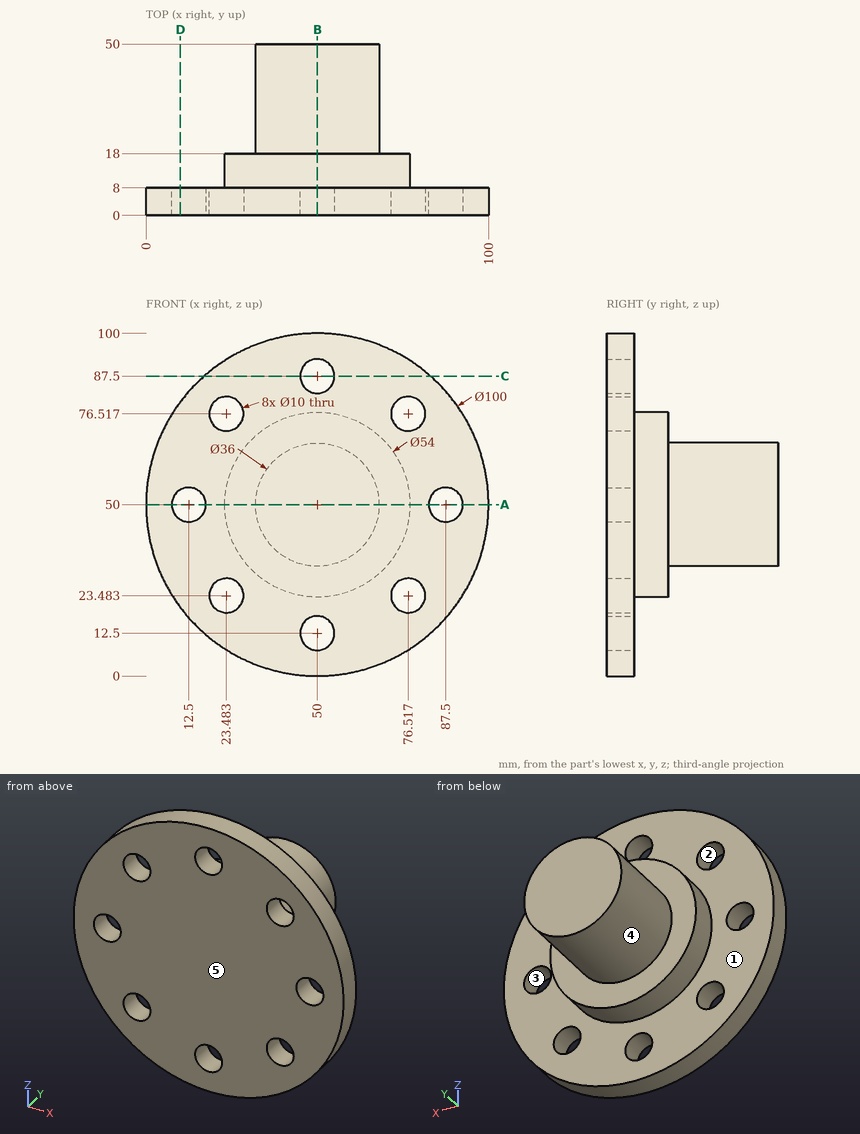
Could you check a few things on this drawing? It's one solid part, dimensions in mm from its lowest x, y, z. A direction names the side the tool comes from. Round coordinates to 2 decimals unless told otherwise and drop trailing zeros. Order: outer loops, then holes, each group sorted by start corner. A loop starts at its lowest first (then second) coordinate and runs counter-clockwise, first axis right, second up. Notation, with made-up numbers: (11.5, 38.5) -> (45.5, 38.5) arc R24 cw to (45.5, 61.5) -> close; hole circle Ø2 at (-24.5, 63.5). An arc over 180 degrees is marked (long way). One line per question, with ' | ' between items.
Q1. We'd pull the mould along X, two halves only. Please class the marked faces 3, 4 and 5: released by +X, released by -X, zero draft, split by the parting line, or undercut.
Computed values:
face 3: undercut | face 4: split by the parting line | face 5: zero draft
Q2. If I drill on line 1 (Y direction, x = 10.5, z = 31); line 2 (Z direction, x = 73, y = 7.5) (1 decimal); line 3 (X direction, y = 5, z = 74.5) (1 decimal), over which ranges is the centre line in solid material (lowest first)? Write a range as from..to.
Computed values:
line 1: 0..8 | line 2: 5.6..19.9, 27..73, 80.1..94.4 | line 3: 6.4..18.9, 28.1..71.9, 81.1..93.6
Q3. Which directions (+Z, -Z, +X, -X, +Y, -Y) give clear straight access to the entire face, cutting with the end or side of a thin tool? Please do the marked faces 1 and 2.
Computed values:
face 1: +Y | face 2: +Y, -Y
Q4. I'm going to push flat-ended pins straight in: pin 1 (6 mm diameter, centred on x = 87.5, z = 50, fed in from -Y); pin 2 (16 mm diameter, centred on x = 50, z = 87.5, fed in from +Y); pin 3 (3 mm diameter, centred on x = 32, y = 38, fed in from +Z) (1 decimal); pin 4 (1.5 mm diameter, centred on x = 17, y = 8.5, fed in from +Z) (1 decimal). Where does each tip first touch, or does it pass through?
Computed values:
pin 1: through | pin 2: y = 8 | pin 3: z = 57.2 | pin 4: z = 88
Q5. If we section it at A-A on z = 50: Write out the boundary of the cut face in (x, y), plus the area to 3 significant figures.
Computed values:
outline: (0, 0) -> (7.5, 0) -> (7.5, 8) -> (0, 8) -> close; (17.5, 0) -> (82.5, 0) -> (82.5, 8) -> (77, 8) -> (77, 18) -> (68, 18) -> (68, 50) -> (32, 50) -> (32, 18) -> (23, 18) -> (23, 8) -> (17.5, 8) -> close; (92.5, 0) -> (100, 0) -> (100, 8) -> (92.5, 8) -> close | area: 2,330 mm²
Q6. If we section it at D-D on x = 10: Write out the boundary of the cut face in (y, z), plus the area to 3 significant figures.
Computed values:
outline: (0, 20) -> (8, 20) -> (8, 45.67) -> (0, 45.67) -> close; (0, 54.33) -> (8, 54.33) -> (8, 80) -> (0, 80) -> close | area: 411 mm²
Q7. If we section it at C-C on z = 87.5: Write out the boundary of the cut face in (x, y).
Computed values:
outline: (16.93, 0) -> (45, 0) -> (45, 8) -> (16.93, 8) -> close; (55, 0) -> (83.07, 0) -> (83.07, 8) -> (55, 8) -> close
Q8. If we section it at B-B on x = 50: Write out the boundary of the cut face in (y, z), plus the area to 3 significant figures.
Computed values:
outline: (0, 0) -> (8, 0) -> (8, 7.5) -> (0, 7.5) -> close; (0, 17.5) -> (8, 17.5) -> (8, 23) -> (18, 23) -> (18, 32) -> (50, 32) -> (50, 68) -> (18, 68) -> (18, 77) -> (8, 77) -> (8, 82.5) -> (0, 82.5) -> close; (0, 92.5) -> (8, 92.5) -> (8, 100) -> (0, 100) -> close | area: 2,330 mm²
